Read the model definition and answer for the solid it produces. Units are mm, in the model's axes. Face numbers are marked on the shaded views. A direction names the side the tool comes from. Coordinates: 2 decimals unless noted, no trailing zeros. Write each loop counter-clockwise with the first axis right and the second up, starting at its lowest first coordinate (ties: lowest second). Pieces come first, ordered by that corner, then holes. Notation, with made-up numbers: (37.5, 51.5) -> (77.5, 51.5) arc R15 ccw to (77.5, 75.5) -> close; hole circle Ø1 at (-21.75, 46.5). An arc over 180 degrees is marked (long way). One line per item, written item: value. Start each with the question number.
1. Find section A-A, the plane z = 10. Write down the section's boundary in (x, y), and give its area (3 significant figures).
2. Given P1, Ø20, axis at y = -2.5, z = 31.65, coming from the +X side; P2, Ø1.5, axis at x = -139.5, y = 28, coming from the -Z side; P3, Ø3, axis at x = -151, y = 13, coming from the +Z side; P4, Ø4, axis at x = -139, z = 30, coming from the -Y side, each flat-ended and moving along its own axis, determine where each tip first touches the part or whether it passes through.
3. Find section D-D, the plane y = 21. Write down the section's boundary in (x, z), and give its area (3 significant figures).
4. For the marked faces 1, 2 and 3, determine the directions among +Z, -Z, +X, -X, +Y, -Y from which every point of the face is accessible in a straight line to the end or side of a thin tool.
5. Consider line 1 along Z through (x, y) = (-160.25, 10); line 2 along Y through (x, z) = (-142, -8.5); line 3 along Y through (x, z) = (-145, 12.5). Determine where each line is inside the solid, lowest interval first.
6. Find section C-C, the plane z = -18. Write down the section's boundary in (x, y).
7. For a pull along Z with two mould halves and no side action, classify the marked faces 4, 5 and 6 as pulls with the +Z half, pulls with the -Z half, needs draft (parallel to the pull), parting line crosses it, or undercut.
8. Find section B-B, the plane x = -151.5. Write down the section's boundary in (y, z), and give its area (3 significant figures).
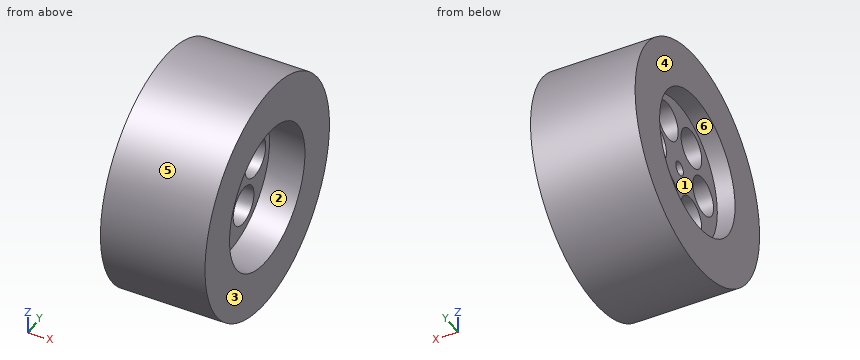
```python
from build123d import *

# Parameters (mm, degrees)
SKETCH004_R     = 66
SKETCH004_R_2   = 4
SKETCH004_R_3   = 11
PAD003_DEPTH    = 29.5
SKETCH005_R     = 40
POCKET001_DEPTH = 20
SKETCH006_R     = 40
POCKET002_DEPTH = 10


with BuildPart() as wheel_right:
    # Sketch004 → Pad003 (new body, symmetric)
    with BuildSketch(Plane.YZ):
        Circle(SKETCH004_R)
        Circle(SKETCH004_R_2, mode=Mode.SUBTRACT)
        with Locations((12.5, -21.650635)):
            Circle(SKETCH004_R_3, mode=Mode.SUBTRACT)
        with Locations((25, 0)):
            Circle(SKETCH004_R_3, mode=Mode.SUBTRACT)
        with Locations((12.5, 21.650635)):
            Circle(SKETCH004_R_3, mode=Mode.SUBTRACT)
        with Locations((-12.5, 21.650635)):
            Circle(SKETCH004_R_3, mode=Mode.SUBTRACT)
        with Locations((-25, 0)):
            Circle(SKETCH004_R_3, mode=Mode.SUBTRACT)
        with Locations((-12.5, -21.650635)):
            Circle(SKETCH004_R_3, mode=Mode.SUBTRACT)
    extrude(amount=PAD003_DEPTH, both=True)

    # Sketch005 (on Face3 of Pad003) → Pocket001 (cut)
    with BuildSketch(Plane(origin=(-29.5, 0, 0), x_dir=(0, 1, 0), z_dir=(-1, 0, 0))):
        Circle(SKETCH005_R)
    extrude(amount=-POCKET001_DEPTH, mode=Mode.SUBTRACT)

    # Sketch006 (on Face3 of Pocket001) → Pocket002 (cut)
    with BuildSketch(Plane.YZ.offset(29.5)):
        Circle(SKETCH006_R)
    extrude(amount=-POCKET002_DEPTH, mode=Mode.SUBTRACT)


with BuildPart() as wheel_right_1:
    # Body003 placement: moved
    add(wheel_right.part.moved(Location((135, 10, 10))))


with BuildPart() as part_mirroring001:
    # Part__Mirroring001: instance of wheel right
    add(wheel_right_1.part.mirror(Plane(origin=(0, 0, 0), x_dir=(0, -1, 0), z_dir=(1, 0, 0))))


solid = part_mirroring001.part
```
Answer block:
1. outline: (-164.5, -56) -> (-105.5, -56) -> (-105.5, -30) -> (-125.5, -30) -> (-125.5, -26) -> (-154.5, -26) -> (-154.5, -30) -> (-164.5, -30) -> close; (-164.5, 50) -> (-154.5, 50) -> (-154.5, 46) -> (-125.5, 46) -> (-125.5, 50) -> (-105.5, 50) -> (-105.5, 76) -> (-164.5, 76) -> close; (-154.5, -4) -> (-125.5, -4) -> (-125.5, 6) -> (-154.5, 6) -> close; (-154.5, 14) -> (-125.5, 14) -> (-125.5, 24) -> (-154.5, 24) -> close
1. area: 3,880 mm2
2. P1: passes through
2. P2: stops at z = -53.71
2. P3: stops at z = 75.98
2. P4: stops at y = -53.5
3. outline: (-164.5, -55.08) -> (-105.5, -55.08) -> (-105.5, -28.46) -> (-125.5, -28.46) -> (-125.5, -22.55) -> (-154.5, -22.55) -> (-154.5, -28.46) -> (-164.5, -28.46) -> close; (-164.5, 48.46) -> (-154.5, 48.46) -> (-154.5, 42.55) -> (-125.5, 42.55) -> (-125.5, 48.46) -> (-105.5, 48.46) -> (-105.5, 75.08) -> (-164.5, 75.08) -> close; (-154.5, -0.75) -> (-125.5, -0.75) -> (-125.5, 20.75) -> (-154.5, 20.75) -> close
3. area: 4,110 mm2
4. face 1: -X
4. face 2: +X
4. face 3: +Z, -Z, +X, +Y, -Y
5. line 1: z = -56 to -30, 50 to 76
5. line 2: y = -53.35 to -13.04, 8.04 to 11.96, 33.04 to 73.35
5. line 3: y = -55.95 to -25.71, -4.29 to 6.88, 13.12 to 24.29, 45.71 to 75.95
6. outline: (-164.5, -49.77) -> (-105.5, -49.77) -> (-105.5, -18.57) -> (-125.5, -18.57) -> (-125.5, -11.48) -> (-154.5, -11.48) -> (-154.5, -18.57) -> (-164.5, -18.57) -> close; (-164.5, 38.57) -> (-154.5, 38.57) -> (-154.5, 31.48) -> (-125.5, 31.48) -> (-125.5, 38.57) -> (-105.5, 38.57) -> (-105.5, 69.77) -> (-164.5, 69.77) -> close; (-154.5, 6.48) -> (-125.5, 6.48) -> (-125.5, 13.52) -> (-154.5, 13.52) -> close
7. face 4: needs draft
7. face 5: parting line crosses it
7. face 6: undercut
8. outline: circle Ø132 at (10, 10); hole circle Ø22 at (-15, 10); hole circle Ø22 at (-2.5, -11.65); hole circle Ø22 at (-2.5, 31.65); hole circle Ø8 at (10, 10); hole circle Ø22 at (22.5, -11.65); hole circle Ø22 at (22.5, 31.65); hole circle Ø22 at (35, 10)
8. area: 11,400 mm2
